Design review of the part shown in the three views and the two pictorial views. Dimensions are in mm from the part's minimum x, y and z. A direction names the side the tool comes from. Coordinates: 2 decimals unless noted, no trailing zeros. Loops run counter-clockwise (first coordinate to the right, second up) from the corner with the lowest first, then second, coordinate; pieces in that order, holes last. Notation, with made-up numbers: (74.5, 17.25) - (94.5, 17.25) arc R20 cw to (94.5, 42.25) - close; hole circle Ø5 at (32.5, 5.5). An arc over 180 degrees is marked (long way). One line per question, with ' | ' between items.
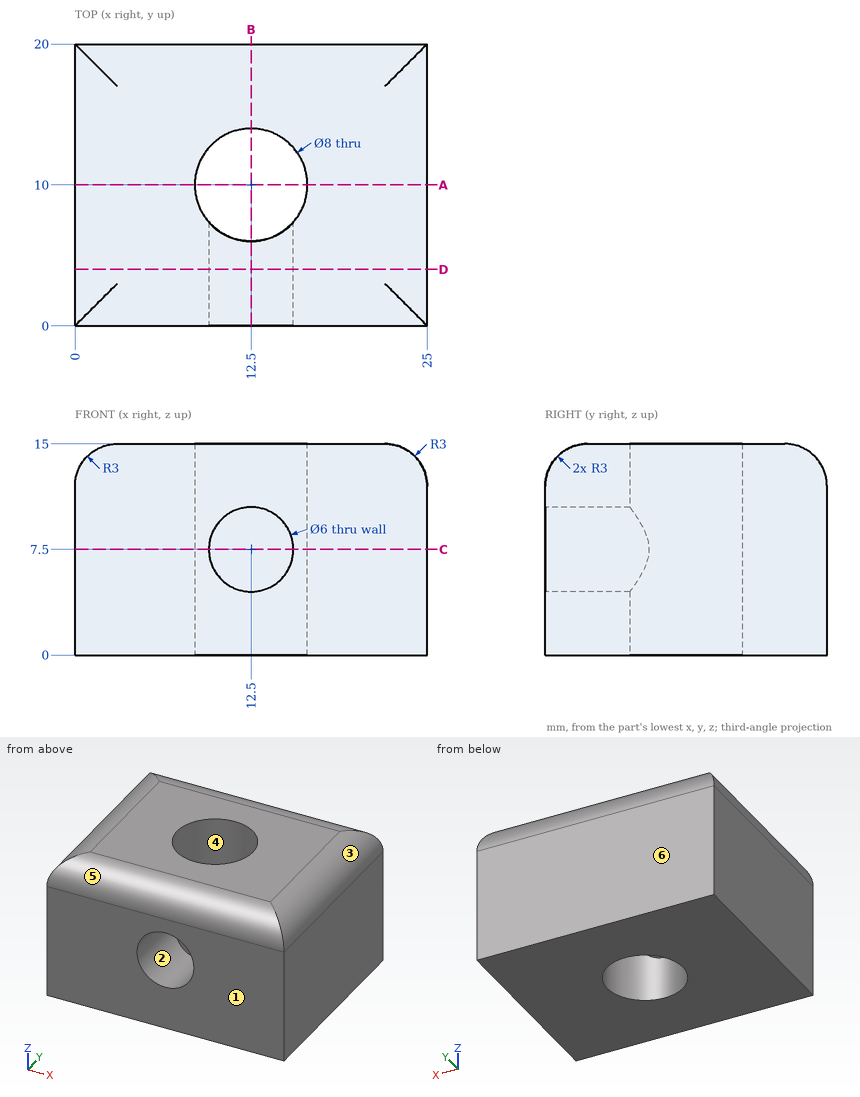
Q1. For pin 1 (5 mm diameter, centred on x = 12.5, y = 10, fed in from +Z); pin 2 (1 mm diameter, centred on x = 20.5, y = 2, fed in from +Z), all flat-tipped, find the tip position at first contact; note any pin that passes through.
Returned:
pin 1: passes through | pin 2: stops at z = 14.96
Q2. Take a section at C-C (z = 7.5). Give the boundary of the cut face in (x, y), plus the area to 3 significant figures.
Returned:
outline: (0, 0) - (9.5, 0) - (9.5, 7.35) arc R4 cw (long way) to (15.5, 7.35) - (15.5, 0) - (25, 0) - (25, 20) - (0, 20) - close | area: 411 mm²
Q3. Take a section at B-B (x = 12.5). Give the boundary of the cut face in (y, z), plus the area to 3 significant figures.
Returned:
outline: (0, 0) - (6, 0) - (6, 4.5) - (0, 4.5) - close; (0, 10.5) - (6, 10.5) - (6, 15) - (3, 15) arc R3 ccw to (0, 12) - close; (14, 0) - (20, 0) - (20, 12) arc R3 ccw to (17, 15) - (14, 15) - close | area: 140 mm²
Q4. To check wall thickness, follow line 1 along Y through (x, z) = (12.5, 2.5); line 2 along Z through (x, y) = (12.5, 3.5); line 3 along Y through (x, z) = (12.5, 5). State the ranges of each line that lie inside material, in increasing order.
Returned:
line 1: y = 0 to 6, 14 to 20 | line 2: z = 0 to 4.5, 10.5 to 15 | line 3: y = 14 to 20
Q5. Take a section at A-A (y = 10). Give the boundary of the cut face in (x, z), plus the area to 3 significant figures.
Returned:
outline: (0, 0) - (8.5, 0) - (8.5, 15) - (3, 15) arc R3 ccw to (0, 12) - close; (16.5, 0) - (25, 0) - (25, 12) arc R3 ccw to (22, 15) - (16.5, 15) - close | area: 251 mm²
Q6. Draft analysis for pull direction Y (two halves, no side actions). For the marked faces 3, 4, 5 and 6, state which applies: +Y half, -Y half, draft (parallel to the pull), parting line (faces both ways), or undercut.
Returned:
face 3: draft | face 4: undercut | face 5: -Y half | face 6: +Y half
Q7. Take a section at D-D (y = 4). Give the boundary of the cut face in (x, z), plus the area to 3 significant figures.
Returned:
outline: (0, 0) - (25, 0) - (25, 12) arc R3 ccw to (22, 15) - (3, 15) arc R3 ccw to (0, 12) - close; hole circle Ø6 at (12.5, 7.5) | area: 343 mm²
Q8. Tool access review of the marked faces 1 and 2: name each direction out of +Z, -Z, +X, -X, +Y, -Y from which nothing blocks a thin tool from reaching the whole face with its end or side.
Returned:
face 1: +Z, -Z, +X, -X, -Y | face 2: -Y
